Input: part model. Units: mm. Frame: model coordinates. A direction names the side the tool comes from. Round coordinates to 2 decimals unless told otherwise and drop trailing zeros. Loops run counter-clockwise (first coordinate to the right, second up) from the corner with the lowest first, then second, coordinate; pieces in that order, holes last. Notation, with made-up numbers: M -23.5,-28 L 0.5,-28 A19 cw 0.5,4 Z; hole C 48.5,-8 d11. An arc over 180 degrees is marked long. Use one line per item in the form item = value. Start each with the question number.
Q1. Access query for faces 1 (the flat face through (25.53, -2.28, -3.88)), 2 (the flat face through (23.5, 5, 0)), 3 (the flat face through (25.528, 2.219, -3.915)), 4 (the flat face through (21.5, 3, -3)). Directions: +Z, -Z, +X, -X, +Y, -Y. A direction counts if a zero-diameter tool reaches every point of the face in a straight line with its end or side. Return the directions, or none.
Q2. First-contact query: P1, Ø1.2, axis at x = 26, z = 0.5, coming from the +Y side; P2, Ø5, axis at x = 14, z = 4, coming from the +Y side; P3, Ø1, axis at x = 6.5, z = 3, coming from the +Y side. Flat tips, straight axial feed; report the tip coordinate or a pass-through.
Q3. Section query C-C, the plane x = 8. Output: boundary loops of the cut face in (y, z).
Q4. Section query D-D, the plane x = 19. Output: boundary loops of the cut face in (y, z), and give its area (3 significant figures).
Q5. Section query A-A, the plane z = 0. Output: boundary loops of the cut face in (x, y).
Q6. Section query B-B, the plane y = 0.75. Output: boundary loops of the cut face in (x, z), and give its area (3 significant figures).
Q7. Ray query, line 1 along X through (y, z) = (-2.5, 2.25); line 2 along X through (y, z) = (-6, 3.5); line 3 along Y through (x, z) = (5.5, 1). Return the intervals inside material, ascending.
```python
from build123d import *

# Parameters (mm, degrees)
BOSS_EXTRUDE1_DEPTH = 4


with BuildPart() as part:
    # Sketch1 → Revolve1 (revolve)
    with BuildSketch(Plane.XY, mode=Mode.PRIVATE) as revolve1_sk:
        Polygon((0, 0), (0, 3), (9.5, 3), (9.5, 4), (21.5, 4), (21.5, 7), (23.5, 7), (23.5, 4.5), (27.5, 4.5), (27.5, 0), align=None)
    revolve(revolve1_sk.sketch.rotate(Axis((0, 0, 0), (1, 0, 0)), 90), axis=Axis((0, 0, 0), (1, 0, 0)))

    # Sketch2 → Boss-Extrude1 (add)
    with BuildSketch(Plane(origin=(27.5, 0, 0), x_dir=(0, 0, -1), z_dir=(1, 0, 0))):
        Polygon((-2.598076211, 4.5), (-5.196152423, 0), (-2.598076211, -4.5), (2.598076211, -4.5), (5.196152423, 0), (2.598076211, 4.5), align=None)
    extrude(amount=-BOSS_EXTRUDE1_DEPTH)


solid = part.part
```
Results found:
q1.face_1 = -Z, +X, -Y
q1.face_2 = +X
q1.face_3 = -Z, +X, +Y
q1.face_4 = -X
q2.P1 = 4.5
q2.P2 = 3.71
q2.P3 = 1.66
q3.outline = C 0,0 d6
q4.outline = C 0,0 d8
q4.area = 50.3 mm²
q5.outline = M 0,-3 L 9.5,-3 L 9.5,-4 L 21.5,-4 L 21.5,-7 L 23.5,-7 L 23.5,-4.5 L 27.5,-4.5 L 27.5,4.5 L 23.5,4.5 L 23.5,7 L 21.5,7 L 21.5,4 L 9.5,4 L 9.5,3 L 0,3 Z
q6.outline = M 0,-2.9 L 9.5,-2.9 L 9.5,-3.93 L 21.5,-3.93 L 21.5,-6.96 L 23.5,-6.96 L 23.5,-4.76 L 27.5,-4.76 L 27.5,4.76 L 23.5,4.76 L 23.5,6.96 L 21.5,6.96 L 21.5,3.93 L 9.5,3.93 L 9.5,2.9 L 0,2.9 Z
q6.area = 215 mm²
q7.line_1 = 9.5 to 27.5
q7.line_2 = 21.5 to 23.5
q7.line_3 = -2.83 to 2.83
